from build123d import *

# Parameters (mm, degrees)
BOSS_EXTRUDE1_DEPTH = 30
CUT_EXTRUDE1_DEPTH  = 13
CUT_EXTRUDE2_START  = -10
CUT_EXTRUDE2_DEPTH  = 10
SKETCH6_R           = 3.175
CUT_EXTRUDE3_DEPTH  = 36.083445782


with BuildPart() as part:
    # Sketch3 → Boss-Extrude1 (new body)
    with BuildSketch(Plane(origin=(0, 0, 0), x_dir=(1, 0, 0), z_dir=(0, 1, 0))):
        with BuildLine():
            Line((37.5, 0), (47.5, 0))
            ThreePointArc((47.5, 0), (45.881476749, 12.293904642), (41.13620668, 23.75))
            Line((41.13620668, 23.75), (32.475952642, 18.75))
            ThreePointArc((32.475952642, 18.75), (36.222218486, 9.705714191), (37.5, 0))
        make_face()
    extrude(amount=BOSS_EXTRUDE1_DEPTH)

    # Sketch4 → Cut-Extrude1 (cut)
    with BuildSketch(Plane(origin=(0, 0, 0), x_dir=(1, 0, 0), z_dir=(0, 1, 0))):
        with BuildLine():
            Line((34.641016151, 20), (38.97114317, 22.5))
            ThreePointArc((38.97114317, 22.5), (43.466662183, 11.64685703), (45, 0))
            Line((45, 0), (40, 0))
            ThreePointArc((40, 0), (38.637033052, 10.352761804), (34.641016151, 20))
        make_face()
    extrude(amount=CUT_EXTRUDE1_DEPTH, mode=Mode.SUBTRACT)

    # Sketch5 → Cut-Extrude2 (cut)
    with BuildSketch(Plane(origin=(0, 30, 0), x_dir=(1, 0, 0), z_dir=(0, 1, 0)).offset(CUT_EXTRUDE2_START)):
        with BuildLine():
            Line((41.13620668, 23.75), (32.475952642, 18.75))
            ThreePointArc((32.475952642, 18.75), (33.632727807, 16.585825883), (34.645482469, 14.350628714))
            Line((34.645482469, 14.350628714), (43.884277794, 18.177463037))
            ThreePointArc((43.884277794, 18.177463037), (42.601455223, 21.008712785), (41.13620668, 23.75))
        make_face()
    cut_extrude2 = extrude(amount=CUT_EXTRUDE2_DEPTH, mode=Mode.SUBTRACT)

    # Mirror1: Cut-Extrude2 across plane
    add(cut_extrude2.mirror(Plane(origin=(0, 0, 0), x_dir=(0.9659258262890681, 0, -0.25881904510252135), z_dir=(0.25881904510252135, 0, 0.9659258262890681))), mode=Mode.SUBTRACT)

    # Sketch6 → Cut-Extrude3 (cut, through all)
    with BuildSketch(Plane(origin=(45.881476749, 0, -12.293904642), x_dir=(-0.25881904510252135, 0, -0.9659258262890682), z_dir=(0.9659258262890681, 0, -0.2588190451025213))):
        with Locations((0, 25)):
            Circle(SKETCH6_R)
    extrude(amount=-CUT_EXTRUDE3_DEPTH, mode=Mode.SUBTRACT)


solid = part.part
Geometry check sheet. Reference: the model listing, model coordinates, mm. A direction names the side the tool comes from. Round coordinates to 2 decimals unless told otherwise and drop trailing zeros. Write each loop counter-clockwise with the first axis right and the second up, starting at its lowest first coordinate (ties: lowest second). Pieces come first, ordered by that corner, then holes.
Item 1: Mould release check, pull along X, two halves, no side actions. Record for faces 1 (the face through (44, 0, -12)), 2 (the face through (42.07, 24.93, -5.54)), 3 (the face through (38.675, 6.409, -10.211)), 4 (the face through (43.424, 6.409, -11.806)): +X half, -X half, draft (parallel to the pull), parting line (faces both ways), or undercut.
Determined:
face 1: draft
face 2: +X half
face 3: undercut
face 4: undercut
Item 2: Material ranges on line 1 along Y through (x, z) = (38.25, -2); line 2 along Y through (x, z) = (39, -14.75); line 3 along X through (y, z) = (3.5, -19), recorded low to high.
Determined:
line 1: y = 0 to 20
line 2: y = 13 to 30
line 3: x = 32.91 to 35.2, 40.79 to 43.53
Item 3: Go/stop test with flat-tipped pins: pin 1 Ø2 at (y, z) = (13, -15.5) entering from -X; pin 2 Ø3 at (y, z) = (12, -6.5) entering from -X; pin 3 Ø2 at (y, z) = (9, -15.5) entering from +X. Record where each tip stops, or that it passes through.
Determined:
pin 1: stops at x = 33.67
pin 2: stops at x = 36.64
pin 3: stops at x = 45.23
Item 4: Section check B-B (z = -17.25). Record the boundary of the cut face in (x, y).
Determined:
outline: (33.3, 0) - (36.09, 0) - (36.09, 13) - (41.56, 13) - (41.56, 0) - (44.26, 0) - (44.26, 30) - (41.65, 30) - (41.65, 20) - (33.3, 20) - close
Item 5: Access from +Z, -Z, +X, -X, +Y, -Y to the whole of each face (thin tool, end or side, straight path). Record for faces 5 (the face through (41, 13, -11)), 6 (the face through (36.186, 11.457, -9.838)), 7 (the face through (38, 20, -19)), 8 (the face through (43, 20, -2)).
Determined:
face 5: -Y
face 6: +Z, -X, +Y, -Y
face 7: -Z, -X, +Y
face 8: +Z, +X, +Y
Item 6: Section check A-A (y = 9). Record the boundary of the cut face in (x, z), plus the area to 3 significant figures.
Determined:
outline: (32.48, -18.75) - (34.64, -20) arc R40 ccw to (40, 0) - (37.5, 0) arc R37.5 cw to start; (38.97, -22.5) - (41.14, -23.75) arc R47.5 ccw to (47.5, 0) - (45, 0) arc R45 cw to start
area: 111 mm2
Item 7: Section check C-C (y = 26). Record the boundary of the cut face in (x, z) (3 decimals).
Determined:
outline: (34.645, -14.351) - (43.884, -18.177) arc R47.5 ccw to (45.009, -15.18) - (35.325, -12.585) arc R37.5 cw to start; (36.885, -6.764) - (46.569, -9.358) arc R47.5 ccw to (47.094, -6.2) - (37.179, -4.895) arc R37.5 cw to start
